Part print with two shaded views. Sizes in mm from the minimum x, y, z corner. Round coordinates to 2 decimals unless told otherwise and drop trailing zeros. Order: outer loops, then holes, each group sorted by start corner. A loop starts at its lowest first (then second) coordinate and runs counter-clockwise, first axis right, second up. Notation, with made-up numbers: M 51,49.25 L 71,49.25 A15 ccw 71,67.25 Z; hole C 76.25,36.25 d3. An arc over 180 degrees is marked long. Return JSON: item names as keys, results as strings. Group by question number.
Item 1: Slice it at D-D on y = 3.85. Give the number of separate pieces and of enclosed holes in the cut face, then the cut area to 3 significant figures.
Item 2: Probe line 1 along Z through (x, y) = (93, 1.8); line 2 along X through (y, z) = (1.35, 13); line 3 along X through (y, z) = (2.45, 20). List the from-to ranges inside material, lowest first.
Item 3: Pin check, flat tips, straight feed: pin 1 Ø8.5 at (x, z) = (107, 13) entering from +Y; pin 2 Ø5.5 at (x, z) = (93, 13) entering from -Y. Stop position of each tip, or through.
Item 4: Slice it at C-C on x = 107. Write the cut outline in (y, z).
Item 5: Slice it at A-A on x = 20. Write the cut outline in (y, z), then the cut area to 3 significant figures.
Item 6: Slice it at B-B on z = 13. Write the cut outline in (x, y), then the cut area to 3 significant figures.
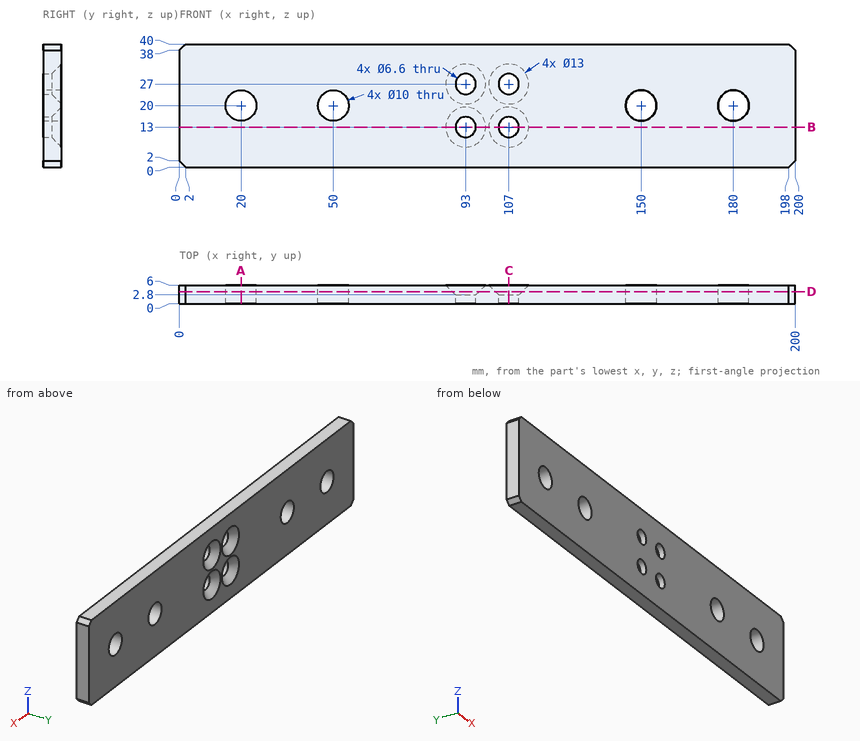
Output values:
{
 "1": {"separate pieces": "1", "enclosed holes": "8", "area": "7,440 mm²"},
 "2": {"line 1": "0 to 9.7, 16.3 to 23.7, 30.3 to 40", "line 2": "0 to 89.7, 96.3 to 103.7, 110.3 to 200", "line 3": "0 to 15, 25 to 45, 55 to 145, 155 to 175, 185 to 200"},
 "3": {"pin 1": "y = 3.75", "pin 2": "through"},
 "4": {"outline": "M 0,0 L 6,0 L 6,6.5 L 2.8,9.7 L 0,9.7 Z; M 0,16.3 L 2.8,16.3 L 6,19.5 L 6,20.5 L 2.8,23.7 L 0,23.7 Z; M 0,30.3 L 2.8,30.3 L 6,33.5 L 6,40 L 0,40 Z"},
 "5": {"outline": "M 0,0 L 6,0 L 6,15 L 0,15 Z; M 0,25 L 6,25 L 6,40 L 0,40 Z", "area": "180 mm²"},
 "6": {"outline": "M 0,0 L 89.7,0 L 89.7,2.8 L 86.5,6 L 0,6 Z; M 96.3,0 L 103.7,0 L 103.7,2.8 L 100.5,6 L 99.5,6 L 96.3,2.8 Z; M 110.3,0 L 200,0 L 200,6 L 113.5,6 L 110.3,2.8 Z", "area": "1,100 mm²"}
}
